Answer from the drawing. Dimensions are ordinates in mm from the lowest x, y and z of the part. Coordinates: 2 decimals unless noted, no trailing zeros. Loops run counter-clockwise (first coordinate to the right, second up) from the corner with the lowest first, then second, coordinate; pieces in that order, holes last. Notation, with made-up numbers: (37, -34) -> (75, -34) arc R17 cw to (75, -11) -> close; hole circle Ø10 at (81.5, 29). An arc over 180 degrees is marked (long way). Answer as CSV lines item,"result".
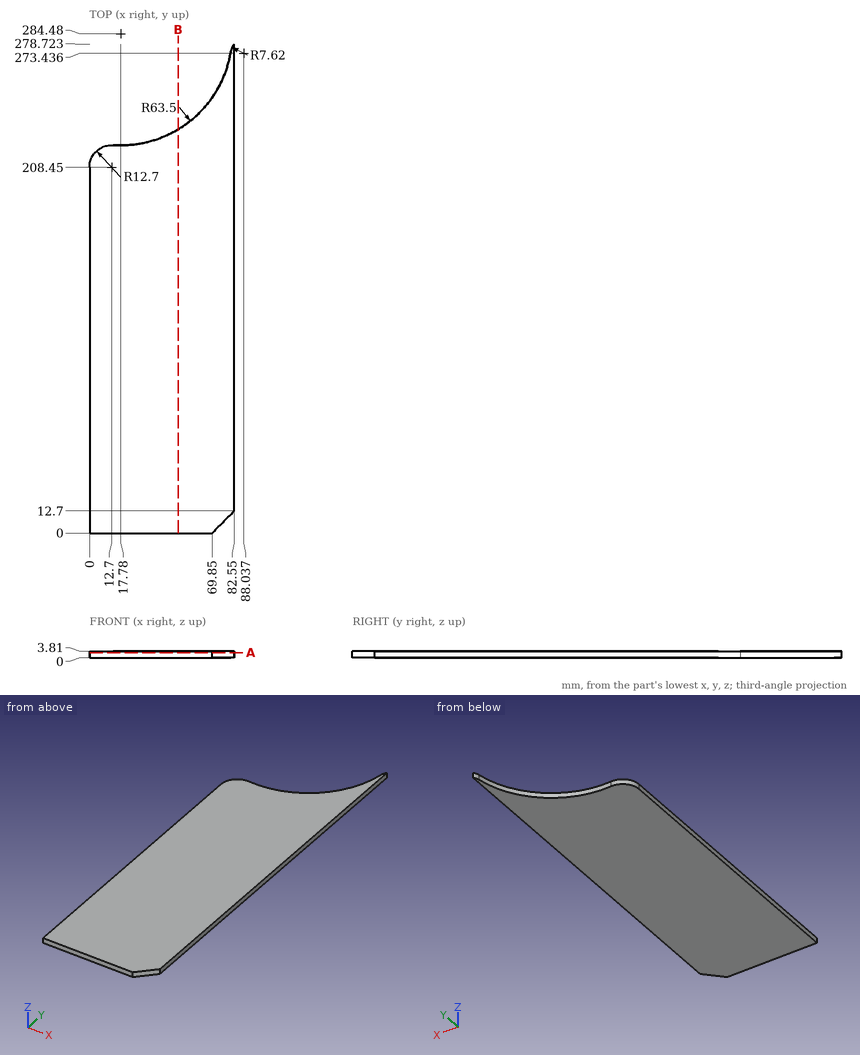
(1) A flat-ended cylindrical pin translates along its axis: pin 1 Ø1 at (x, z) = (54, 1) entering from -Y. Find the tip coordinate at first contact, or state that the pin passes through.
Computed values:
pin 1,"y = 0"
(2) A cutting plane is placed at B-B, the plane x = 50.5. Write down the section's boundary in (y, z).
Computed values:
outline,"(0, 0) -> (230.06, 0) -> (230.06, 3.81) -> (0, 3.81) -> close"
(3) A cutting plane is placed at A-A, the plane z = 3. Write down the section's boundary in (x, y).
Computed values:
outline,"(0, 0) -> (69.85, 0) -> (82.55, 12.7) -> (82.55, 278.72) arc R7.62 ccw to (80.51, 274.62) arc R63.5 cw to (13.55, 221.12) arc R12.7 ccw to (0, 208.45) -> close"
(4) Consider line 1 along Y through (x, z) = (13, 1.95) (1 decimal); line 2 along Y through (x, z) = (18, 1.55). Determine where each line is inside the solid, lowest interval first.
Computed values:
line 1,"0 to 221.1"
line 2,"0 to 220.98"
